```python
from build123d import *

# Parameters (mm, degrees)
F0_W     = 158.75
F0_H     = 82.55
F1_DEPTH = 25.4
F2_W     = 152.4
F2_H     = 76.2
F3_DEPTH = 22.225
F4_ANGLE = 180


with BuildPart() as f1:
    # F0 (on Top) → F1 (new body)
    with BuildSketch(Plane.XY):
        Rectangle(F0_W, F0_H)
    extrude(amount=F1_DEPTH)

    # F2 (on Top) → F3 (cut)
    with BuildSketch(Plane.XY):
        Rectangle(F2_W, F2_H)
    extrude(amount=F3_DEPTH, mode=Mode.SUBTRACT)


with BuildPart() as f1_1:
    # F4: moved
    add(f1.part.rotate(Axis((79.375, 0, 0), (0, -1, 0)), F4_ANGLE))


solid = f1_1.part
```
Can you work these out from the model? Positions are in its coordinate system, mm. A direction names the side the tool comes from. Give positions to 0.01 mm unless a question says otherwise; leave off trailing zeros. Order: outer loops, then holes, each group sorted by start corner. A loop starts at its lowest first (then second) coordinate and runs counter-clockwise, first axis right, second up. Notation, with made-up numbers: M 31,28 L 53,28 A30 ccw 53,67 Z; hole C 13.5,-3.5 d7. An arc over 180 degrees is marked long. One line per item, written item: value.
1) We'd pull the mould along X, two halves only. Please class faces 1 (the face through (238.125, -1, -13)), 2 (the face through (79.375, -1, -13)), 3 (the face through (160, -38.1, -11)), 4 (the face through (160, 38.1, -11)): released by +X, released by -X, zero draft, split by the parting line, or undercut.
Answer sheet:
face 1: released by +X
face 2: released by -X
face 3: undercut
face 4: undercut
2) On a 3-axis mill with a long thin cutter (end or side, diameter ignored), from which of +Z, -Z, +X, -X, +Y, -Y can I reach the whole of each face in a straight line? I mean faces 5 (the face through (160, 1, -22.225)), 6 (the face through (160, 1, -25.4)). Say none if no direction works.
Answer sheet:
face 5: +Z
face 6: -Z, +X, -X, +Y, -Y
3) Please list where these lines run through material, in increasing order: line 1 along Y through (x, z) = (200.5, -5.5) (3 decimals); line 2 along X through (y, z) = (9, -14.75) (3 decimals); line 3 along Z through (x, y) = (139, -36) (3 decimals).
Answer sheet:
line 1: y = -41.275 to -38.1, 38.1 to 41.275
line 2: x = 79.375 to 82.55, 234.95 to 238.125
line 3: z = -25.4 to -22.225
4) I want a section at C-C, the plane x = 142. List the corners of the cut face in (y, z) for me (3 decimals), plus the area to 3 significant figures.
Answer sheet:
outline: M -41.275,-25.4 L 41.275,-25.4 L 41.275,0 L 38.1,0 L 38.1,-22.225 L -38.1,-22.225 L -38.1,0 L -41.275,0 Z
area: 403 mm^2
5) I want a section at A-A, the plane z = -17. List the corners of the cut face in (x, y) for me (3 decimals).
Answer sheet:
outline: M 79.375,-41.275 L 238.125,-41.275 L 238.125,41.275 L 79.375,41.275 Z; hole M 82.55,-38.1 L 234.95,-38.1 L 234.95,38.1 L 82.55,38.1 Z
6) I want a section at B-B, the plane y = 6. List the corners of the cut face in (x, z) for me (3 decimals), plus the area to 3 significant figures.
Answer sheet:
outline: M 79.375,-25.4 L 238.125,-25.4 L 238.125,0 L 234.95,0 L 234.95,-22.225 L 82.55,-22.225 L 82.55,0 L 79.375,0 Z
area: 645 mm^2
7) For P1, Ø12, axis at x = 127, y = -32, coming from the +Z side (3 decimals), with a flat end and sliding along its axis, tell me the tip position at first contact or that it passes through.
Answer sheet:
P1: stops at z = -22.225
